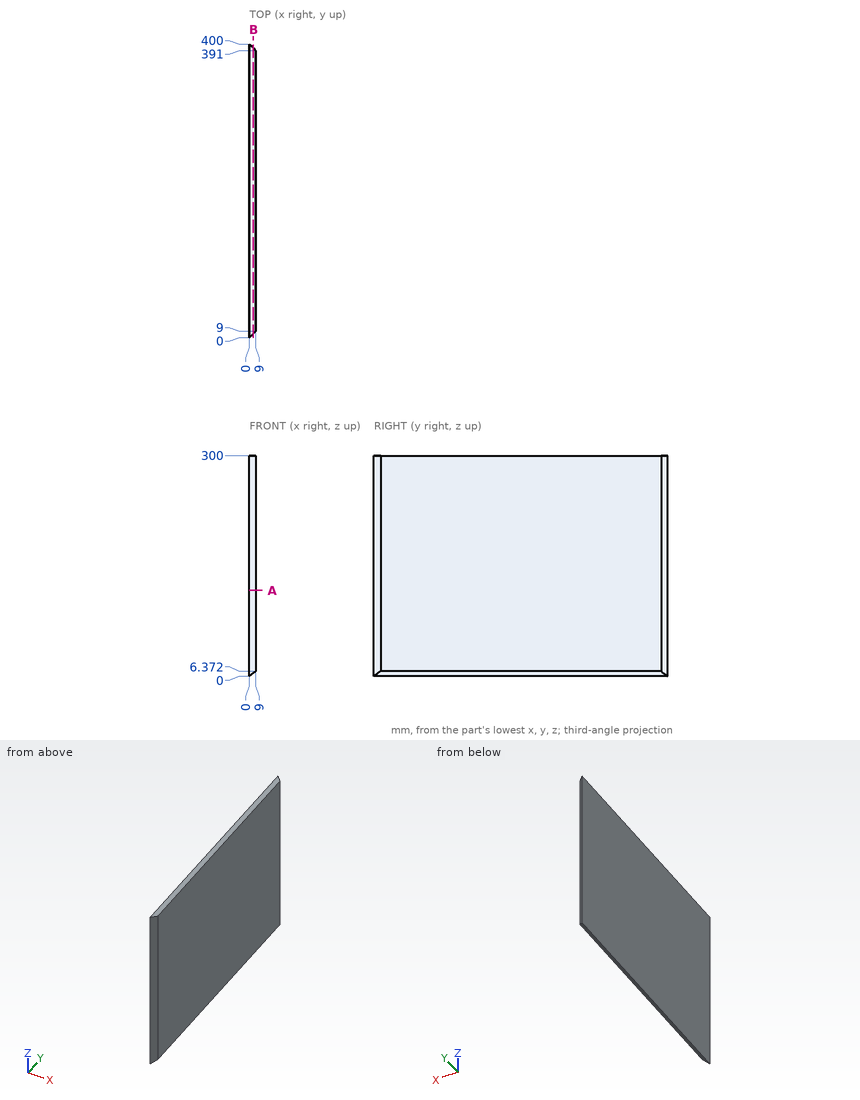
Input: dimensioned drawing with shaded views. Units: mm. Origin: part minimum x, y, z. Round coordinates to 2 decimals unless told otherwise and drop trailing zeros. Order: outer loops, then holes, each group sorted by start corner. A loop starts at its lowest first (then second) coordinate and runs counter-clockwise, first axis right, second up. Notation, with made-up numbers: (-23.5, 80.5) - (-1.5, 80.5) arc R7 cw to (-1.5, 86.5) - close; hole circle Ø9 at (59.25, 31). An arc over 180 degrees is marked (long way). Write item = value, one per line. Start each with the question number.
Q1. Pin query (flat end, axial travel): pin 1 (5 mm diameter, centred on x = 6.5, z = 237.5, fed in from -Y). Return the tip coordinate at first contact, or that it passes through.
Q2. Ray query, line 1 (Y direction, x = 3, z = 42.5); line 2 (Y direction, x = 1.5, z = 46); line 3 (Z direction, x = 7.25, y = 297.5) (1 decimal). Return the intervals inside material, ascending. Write a range as from..to.
Q3. Cut plane B-B on x = 5.5. Return the cut outline in (y, z), and give its area (3 significant figures).
Q4. Cut plane A-A on z = 116.5. Return the cut outline in (x, y), and give its area (3 significant figures).
Outcome:
q1.pin_1 = 4
q2.line_1 = 3..397
q2.line_2 = 1.5..398.5
q2.line_3 = 5.1..300
q3.outline = (5.5, 3.89) - (394.5, 3.89) - (394.5, 300) - (5.5, 300) - close
q3.area = 115,000 mm^2
q4.outline = (0, 0) - (9, 9) - (9, 391) - (0, 400) - close
q4.area = 3,520 mm^2
